```python
from build123d import *

# Parameters (mm, degrees)
SKETCH1_W           = 288
SKETCH1_H           = 250
BOSS_EXTRUDE1_DEPTH = 6
CUT_EXTRUDE1_DEPTH  = 7
LPATTERN4_COUNT     = 6
LPATTERN4_PITCH     = 48


with BuildPart() as part:
    # Sketch1 → Boss-Extrude1 (new body)
    with BuildSketch(Plane.XY):
        with Locations((144, 125)):
            Rectangle(SKETCH1_W, SKETCH1_H)
    extrude(amount=BOSS_EXTRUDE1_DEPTH)

    # Sketch2 → Cut-Extrude1 (cut, through all)
    with BuildSketch(Plane.XY.offset(6)):
        with BuildLine():
            Line((16.5, 24), (16.5, 226))
            ThreePointArc((16.5, 226), (24, 233.5), (31.5, 226))
            Line((31.5, 226), (31.5, 24))
            ThreePointArc((31.5, 24), (24, 16.5), (16.5, 24))
        make_face()
    cut_extrude1 = extrude(amount=-CUT_EXTRUDE1_DEPTH, mode=Mode.SUBTRACT)

    # LPattern4: Cut-Extrude1 ×6
    with Locations(*[(i * LPATTERN4_PITCH, 0, 0) for i in range(1, LPATTERN4_COUNT)]):
        add(cut_extrude1, mode=Mode.SUBTRACT)


solid = part.part
```
Input: part model. Units: mm. Frame: model coordinates. Round coordinates to 2 decimals unless told otherwise and drop trailing zeros. Loops run counter-clockwise (first coordinate to the right, second up) from the corner with the lowest first, then second, coordinate; pieces in that order, holes last. Notation, with made-up numbers: (-5, -18.75) - (6, -18.75) arc R21 cw to (6, 20.25) - close; hole circle Ø6 at (75, -19.5). An arc over 180 degrees is marked (long way). One line per item, written item: value. Start each with the question number.
(1) Section B-B, the plane x = 216. Return loops of the section in (y, z), plus the area to 3 significant figures.
(2) Draft query along X for faces 1 (the cylindrical face through (167.84, 233.5, 3.04)), 2 (the flat face through (142, 250, 3)), 3 (the flat face through (0, 123, 3)). Return one class per face: +X half, -X half, draft (parallel to the pull), parting line (faces both ways), or undercut.
(3) Section C-C, the plane z = 1.5. Return loops of the section in (x, y), plus the area to 3 significant figures.
(4) Section A-A, the plane y = 210. Return loops of the section in (x, z), plus the area to 3 significant figures.
(5) Section D-D, the plane x = 170.5. Return loops of the section in (y, z).
(6) Ray query, line 1 (Y direction, x = 260, z = 5.1); line 2 (Y direction, x = 122, z = 5). Return the intervals inside material, ascending. Write a range as [from, to].
(7) Contact query for a flat-ended pin moving along its axis: P1, Ø1.5, axis at y = 38, z = 4.5, coming from the -X side. Output: stop coordinate, or through.
Results below:
1. outline: (0, 0) - (16.5, 0) - (16.5, 6) - (0, 6) - close; (233.5, 0) - (250, 0) - (250, 6) - (233.5, 6) - close
1. area: 198 mm^2
2. face 1: undercut
2. face 2: draft
2. face 3: -X half
3. outline: (0, 0) - (288, 0) - (288, 250) - (0, 250) - close; hole (16.5, 24) arc R7.5 ccw to (31.5, 24) - (31.5, 226) arc R7.5 ccw to (16.5, 226) - close; hole (64.5, 24) arc R7.5 ccw to (79.5, 24) - (79.5, 226) arc R7.5 ccw to (64.5, 226) - close; hole (112.5, 24) arc R7.5 ccw to (127.5, 24) - (127.5, 226) arc R7.5 ccw to (112.5, 226) - close; hole (160.5, 24) arc R7.5 ccw to (175.5, 24) - (175.5, 226) arc R7.5 ccw to (160.5, 226) - close; hole (208.5, 24) arc R7.5 ccw to (223.5, 24) - (223.5, 226) arc R7.5 ccw to (208.5, 226) - close; hole (256.5, 24) arc R7.5 ccw to (271.5, 24) - (271.5, 226) arc R7.5 ccw to (256.5, 226) - close
3. area: 52,800 mm^2
4. outline: (0, 0) - (16.5, 0) - (16.5, 6) - (0, 6) - close; (31.5, 0) - (64.5, 0) - (64.5, 6) - (31.5, 6) - close; (79.5, 0) - (112.5, 0) - (112.5, 6) - (79.5, 6) - close; (127.5, 0) - (160.5, 0) - (160.5, 6) - (127.5, 6) - close; (175.5, 0) - (208.5, 0) - (208.5, 6) - (175.5, 6) - close; (223.5, 0) - (256.5, 0) - (256.5, 6) - (223.5, 6) - close; (271.5, 0) - (288, 0) - (288, 6) - (271.5, 6) - close
4. area: 1,190 mm^2
5. outline: (0, 0) - (16.93, 0) - (16.93, 6) - (0, 6) - close; (233.07, 0) - (250, 0) - (250, 6) - (233.07, 6) - close
6. line 1: [0, 17.66], [232.34, 250]
6. line 2: [0, 16.77], [233.23, 250]
7. P1: x = 0
